Source: CAD feature listing. Evaluate the final solid. Frame: model axes, mm. Give positions to 0.01 mm unless a question says otherwise; leave off trailing zeros. Order: outer loops, then holes, each group sorted by start corner. A loop starts at its lowest first (then second) coordinate and runs counter-clockwise, first axis right, second up. Notation, with made-up numbers: M -39,87.25 L -7,87.25 A11 cw -7,105.25 Z; hole C -7.75,10 d6. An arc over 180 degrees is marked long. Return JSON: item names as keys, results as strings.
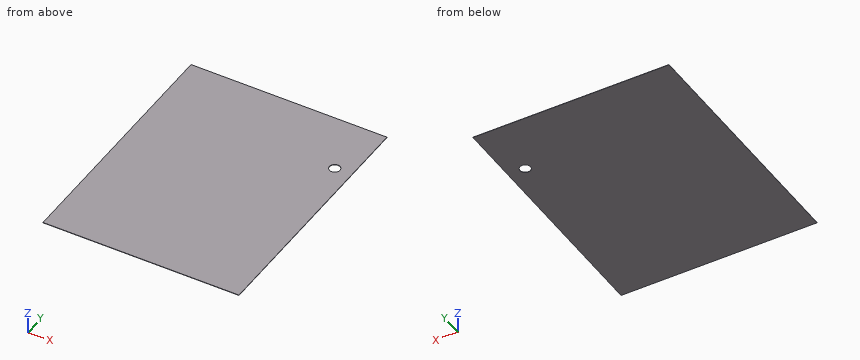
Autodesk Inventor part; units mm, degrees
ref_plane "YZ Plane" through (0, 0, 0) normal (1, 0, 0) x (0, 1, 0)
ref_plane "XZ Plane" through (0, 0, 0) normal (0, 1, 0) x (-1, 0, 0)
ref_plane "XY Plane" through (0, 0, 0) normal (0, 0, 1) x (1, 0, 0)
sketch "Sketch6" plane through (0, 0, 0) normal (0, 0, 1) x (1, 0, 0)
  line L0 (739.5, 947.5) -> (-739.5, 947.5)
  line L1 (-739.5, 947.5) -> (-739.5, -947.5)
  line L2 (-739.5, -947.5) -> (739.5, -947.5)
  line L3 (739.5, -947.5) -> (739.5, 947.5)
  line L4 (739.5, 947.5) -> (-739.5, -947.5) construction
  line L5 (-739.5, 947.5) -> (739.5, -947.5) construction
  point P0 (0, 0)
  dimension "d40" = 1479
  dimension "d41" = 1895
extrude "Plate5" add sketch "Sketch6" along normal blind 3
sketch "Sketch7" plane through (0, 0, 0) normal (0, 0, -1) x (-1, 0, 0)
  line L0 (-714.5, 922.5) -> (-514.5, 922.5) construction
  line L1 (-514.5, 922.5) -> (-514.5, 907.5) construction
  line L2 (-514.5, 907.5) -> (-714.5, 907.5) construction
  line L3 (-714.5, 907.5) -> (-714.5, 922.5) construction
  line L4 (-739.5, 947.5) -> (739.5, 947.5)
  line L5 (-739.5, -947.5) -> (-739.5, 947.5)
  point P0 (0, 0)
  dimension "d43" = 200
  dimension "d44" = 15
  dimension "d45" = 25
  dimension "d46" = 25
mark "Mark1"
sketch "Sketch8" plane through (739.5, 947.5, 0) normal (0, 0, -1) x (-1, 0, 0)
  circle A0 centre (129, -450) radius 40
  line L0 (1479, 0) -> (1479, -1895)
  line L1 (0, 0) -> (1479, 0)
  point P0 (739.5, -947.5)
  dimension "d47" = 80
  dimension "d48" = 1350
  dimension "d49" = 450
extrude "Extrusion3" cut sketch "Sketch8" against normal up to surface (3 mm away)
equation "\"d42\" = Thickness"
equation "\"BendReliefWidth\" = Thickness"
equation "\"BendReliefDepth\" = 0.5 * Thickness"
equation "\"CornerReliefSize\" = 4 * Thickness"
equation "\"MinimumRemnant\" = 2 * Thickness"
equation "\"TransitionRadius\" = BendRadius"
equation "\"JacobiRadiusSize\" = BendRadius"
equation "\"GapSize\" = Thickness"
properties part number "BSH 046 back" material "09g2s"
1. First-contact query: pin 1 (4 mm diameter, centred on x = -409.5, y = 211, fed in from -Z). Flat tip, straight axial feed; report the tip coordinate or a pass-through.
Evaluation:
{"pin 1": "stops at z = 0"}
2. Section query B-B (y = 497.5). Return loops of the section in (x, z), then the cut area to 3 significant figures.
Evaluation:
{"outline": "M -739.5,0 L 570.5,0 L 570.5,3 L -739.5,3 Z; M 650.5,0 L 739.5,0 L 739.5,3 L 650.5,3 Z", "area": "4,200 mm^2"}
3. Ray query, probe 1 along Y at (x, z) = (610.5, 1.9); probe 2 along Y at (x, z) = (625.5, 1.5). Return the intervals inside material, ascending.
Evaluation:
{"probe 1": "y = -947.5 to 457.5, 537.5 to 947.5", "probe 2": "y = -947.5 to 460.42, 534.58 to 947.5"}
4. Section query A-A (x = 610.5). Return loops of the section in (y, z), then the cut area to 4 significant figures.
Evaluation:
{"outline": "M -947.5,0 L 457.5,0 L 457.5,3 L -947.5,3 Z; M 537.5,0 L 947.5,0 L 947.5,3 L 537.5,3 Z", "area": "5,445 mm^2"}
